from build123d import *

# Parameters (mm, degrees)
EXTRUDE_THIN1_DEPTH     = 300
CUT_EXTRUDE1_DEPTH      = 341.036762718
CUT_EXTRUDE1_DEPTH_BACK = 341.036762718
BOSS_EXTRUDE1_REACH     = 398.989
CUT_EXTRUDE2_REACH      = 342.037
FILLET1_R               = 5


with BuildPart() as part:
    # Sketch1 → Extrude-Thin1 (new body)
    with BuildSketch(Plane.XY):
        with BuildLine():
            Line((125, 100), (125, 15))
            ThreePointArc((125, 15), (120.606601718, 4.393398282), (110, 0))
            Line((110, 0), (-110, 0))
            ThreePointArc((-110, 0), (-120.606601718, 4.393398282), (-125, 15))
            Line((-125, 15), (-125, 100))
            Line((-125, 100), (-115, 100))
            Line((-115, 100), (-115, 15))
            ThreePointArc((-115, 15), (-113.535533906, 11.464466094), (-110, 10))
            Line((-110, 10), (110, 10))
            ThreePointArc((110, 10), (113.535533906, 11.464466094), (115, 15))
            Line((115, 15), (115, 100))
            Line((115, 100), (125, 100))
        make_face()
    extrude(amount=-EXTRUDE_THIN1_DEPTH)

    # Sketch2 → Cut-Extrude1 (cut, two sides: drawn at the far end of the back side and taken through both)
    with BuildSketch(Plane.ZY.offset(-CUT_EXTRUDE1_DEPTH_BACK)):
        with BuildLine():
            ThreePointArc((-75, 80), (-36.109127035, 63.890872965), (-20, 25))
            ThreePointArc((-20, 25), (-15, 20), (-10, 25))
            ThreePointArc((-10, 25), (-29.038059223, 70.961940777), (-75, 90))
            ThreePointArc((-75, 90), (-80, 85), (-75, 80))
        make_face()
    extrude(amount=CUT_EXTRUDE1_DEPTH + CUT_EXTRUDE1_DEPTH_BACK, mode=Mode.SUBTRACT)

    # Boss-Extrude1: up to this face of the body (flat: up to its plane)
    boss_extrude1_end = Plane(part.part.faces().sort_by_distance((-115, 57.288670869, -154.695150869))[0])
    # Sketch3 → Boss-Extrude1 (add, up to the picked face)
    with BuildSketch(Plane.ZY.offset(-115), mode=Mode.PRIVATE) as boss_extrude1_sk1:
        Polygon((-300, 80), (-280, 80), (-280, 74), (-294, 74), (-294, 10), (-300, 10), align=None)
    boss_extrude1_tool1 = split(extrude(boss_extrude1_sk1.sketch, amount=BOSS_EXTRUDE1_REACH, mode=Mode.PRIVATE), bisect_by=boss_extrude1_end, keep=Keep.BOTH, mode=Mode.PRIVATE)
    add(boss_extrude1_tool1.solids().sort_by(Axis((115, 50.333333, -295.333333), (-1, 0, 0)))[0])

    # Sketch4 → Cut-Extrude2 (cut, up to next)
    with BuildSketch(Plane(origin=(0, 0, -300), x_dir=(-1, 0, 0), z_dir=(0, 0, -1)), mode=Mode.PRIVATE) as cut_extrude2_sk1:
        with BuildLine():
            Line((-100, 60), (100, 60))
            ThreePointArc((100, 60), (103.535533906, 58.535533906), (105, 55))
            Line((105, 55), (105, 25))
            ThreePointArc((105, 25), (103.535533906, 21.464466094), (100, 20))
            Line((100, 20), (-100, 20))
            ThreePointArc((-100, 20), (-103.535533906, 21.464466094), (-105, 25))
            Line((-105, 25), (-105, 55))
            ThreePointArc((-105, 55), (-103.535533906, 58.535533906), (-100, 60))
        make_face()
    cut_extrude2_tool1 = extrude(cut_extrude2_sk1.sketch, amount=-CUT_EXTRUDE2_REACH, mode=Mode.PRIVATE) & part.part
    add(cut_extrude2_tool1.solids().sort_by_distance((0, 40, -300))[0], mode=Mode.SUBTRACT)

    # Fillet1
    fillet1_edges = [part.edges().sort_by_distance(p)[0] for p in [
        (120, 100, 0),
        (-120, 100, 0),
        (120, 100, -300),
        (0, 80, -300),
        (-120, 100, -300),
    ]]
    fillet(fillet1_edges, radius=FILLET1_R)


solid = part.part
Verification items for the finished model (mm, model axes). A direction names the side the tool comes from. Give positions to 0.01 mm unless a question says otherwise; leave off trailing zeros. Write each loop counter-clockwise with the first axis right and the second up, starting at its lowest first coordinate (ties: lowest second). Pieces come first, ordered by that corner, then holes. Notation, with made-up numbers: M -1.75,31 L 10.25,31 A20 cw 10.25,45 Z; hole C 26.25,-15 d1. An arc over 180 degrees is marked long. Put each result on its own line as item: value. Start each with the question number.
1. Draft check along Y on faces 4 (the face through (-120, 20, -15)), 5 (the face through (120, 100, -148)), 6 (the face through (125, 58, -148)). Enter one of: +Y half, -Y half, draft (parallel to the pull), parting line (faces both ways), or undercut.
2. Go/stop test with flat-tipped pins: pin 1 Ø1.8 at (x, y) = (-27, 78) entering from +Z; pin 2 Ø6.5 at (x, z) = (31, -296) entering from +Y; pin 3 Ø12 at (x, y) = (84.5, 64) entering from +Z; pin 4 Ø12 at (x, y) = (5.5, 21) entering from -Z. Record where each tip stops, or that it passes through.
3. Section check D-D (z = -148). Record the cut outline in (x, y).
4. Section check A-A (z = -15). Record the cut outline in (x, y), and give its area (3 significant figures).
5. Section check B-B (y = 85). Record the cut outline in (x, z), and give its area (3 significant figures).
6. Section check C-C (x = -25.5). Record the cut outline in (y, z).
7. Scan lines: line 1 along X through (y, z) = (25, -97); line 2 along Y through (x, z) = (56.5, -279.5); line 3 along Z through (x, y) = (13, 15.5). Record each from-to range of solid material in increasing order. Write a range as [from, to].
8. Set-up check for faces 1 (the face through (9, 63, -294)), 2 (the face through (-120.49, 4.28, -147.9)), 3 (the face through (-119.93, 64.316, -36.539)): record each of +Z, -Z, +X, -X, +Y, -Y from which the full face is reachable in a straight line by a thin tool's end or side.
Answer list:
1. face 4: undercut
1. face 5: +Y half
1. face 6: draft
2. pin 1: z = -280
2. pin 2: y = 80
2. pin 3: z = -294
2. pin 4: z = -300
3. outline: M -125,15 A15 ccw -110,0 L 110,0 A15 ccw 125,15 L 125,100 L 115,100 L 115,15 A5 cw 110,10 L -110,10 A5 cw -115,15 L -115,100 L -125,100 Z
4. outline: M -125,15 A15 ccw -110,0 L 110,0 A15 ccw 125,15 L 125,20 L 115,20 L 115,15 A5 cw 110,10 L -110,10 A5 cw -115,15 L -115,20 L -125,20 Z; M -125,50 L -115,50 L -115,100 L -125,100 Z; M 115,50 L 125,50 L 125,100 L 115,100 Z
4. area: 3,610 mm2
5. outline: M -125,-300 L -115,-300 L -115,-80 L -125,-80 Z; M -125,-50 L -115,-50 L -115,0 L -125,0 Z; M 115,-300 L 125,-300 L 125,-80 L 115,-80 Z; M 115,-50 L 125,-50 L 125,0 L 115,0 Z
5. area: 5,400 mm2
6. outline: M 0,-300 L 20,-300 L 20,-294 L 10,-294 L 10,0 L 0,0 Z; M 60,-300 L 75,-300 A5 ccw 80,-295 L 80,-280 L 74,-280 L 74,-294 L 60,-294 Z
7. line 1: [-125, -115], [115, 125]
7. line 2: [0, 10]
7. line 3: [-300, -294]
8. face 1: +Z
8. face 2: +Z, -Z, -X, -Y
8. face 3: +X, -X
